from build123d import *

# Parameters (mm, degrees)
CROQUIS1_R              = 1.75
CROQUIS1_R_2            = 1.5
SALIENTE_EXTRUIR1_DEPTH = 2.5


with BuildPart() as part:
    # Croquis1 → Saliente-Extruir1 (new body)
    with BuildSketch(Plane(origin=(0, 0, 0), x_dir=(0, 0, -1), z_dir=(1, 0, 0))):
        with BuildLine():
            Line((95, 10), (90, 10))
            ThreePointArc((90, 10), (64.751798433, 28.463425825), (33.494108419, 27.311648705))
            ThreePointArc((33.494108419, 27.311648705), (20.033827629, 26.787261985), (6.785305839, 29.222587577))
            ThreePointArc((6.785305839, 29.222587577), (-24.970289012, 16.62782808), (-24.346472536, -17.528527464))
            ThreePointArc((-24.346472536, -17.528527464), (-24.321884003, -22.514223272), (-20, -25))
            ThreePointArc((-20, -25), (34.355278896, -56.609528466), (95, -40))
            Line((95, -40), (95, -35))
            Line((95, -35), (100, -35))
            Line((100, -35), (100, 5))
            Line((100, 5), (95, 5))
            Line((95, 5), (95, 10))
        make_face()
        with Locations((-12.730077402, 5.654698909)):
            Circle(CROQUIS1_R, mode=Mode.SUBTRACT)
        with Locations((-5.658477353, 12.726298958)):
            Circle(CROQUIS1_R, mode=Mode.SUBTRACT)
        with Locations((26.870057685, -19.798989873)):
            Circle(CROQUIS1_R, mode=Mode.SUBTRACT)
        with Locations((19.797157185, -26.871890373)):
            Circle(CROQUIS1_R, mode=Mode.SUBTRACT)
        with Locations((-20, -20)):
            Circle(CROQUIS1_R, mode=Mode.SUBTRACT)
        with Locations((90, -6.821183735)):
            Circle(CROQUIS1_R_2, mode=Mode.SUBTRACT)
        with Locations((90, -24.395183951)):
            Circle(CROQUIS1_R_2, mode=Mode.SUBTRACT)
        with Locations((44.87119885, -46.048776814)):
            Circle(CROQUIS1_R_2, mode=Mode.SUBTRACT)
        with Locations((44.87119885, 24.012524519)):
            Circle(CROQUIS1_R_2, mode=Mode.SUBTRACT)
        Polygon((-14.142135624, 0), (14.142135624, -28.284271247), (20.150710576, -22.275696296), (24.393351263, -26.518336983), (26.516504294, -24.395183951), (22.273863607, -20.152543264), (28.284271247, -14.142135624), (0, 14.142135624), (-6.01040764, 8.131727984), (-10.253048327, 12.374368671), (-12.374368671, 10.253048327), (-8.131727984, 6.01040764), align=None, mode=Mode.SUBTRACT)
    extrude(amount=SALIENTE_EXTRUIR1_DEPTH)


solid = part.part
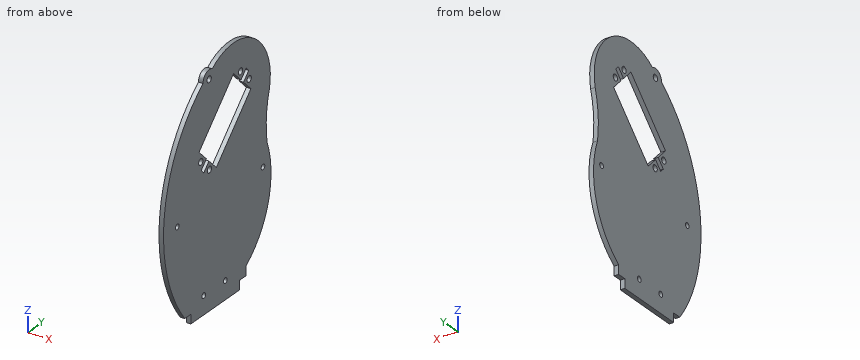
Read the model definition and answer for the solid it produces. Units are mm, in the model's axes. Coordinates: 2 decimals unless noted, no trailing zeros. Order: outer loops, then holes, each group sorted by start corner. A loop starts at its lowest first (then second) coordinate and runs counter-clockwise, first axis right, second up. Notation, with made-up numbers: M -30,-22.75 L 13,-22.75 A15 cw 13,4.25 Z; hole C -28.5,84 d9. An arc over 180 degrees is marked long. Put each result on its own line as item: value. Start each with the question number.
Item 1: Given pin 1 Ø3 at (y, z) = (-20, 20) entering from +X; pin 2 Ø0.8 at (x, y) = (1, -36.5) entering from -Z; pin 3 Ø0.8 at (x, z) = (0.5, -93) entering from +Y; pin 4 Ø1.2 at (x, z) = (0.5, -97.5) entering from -Y, each flat-ended and moving along its own axis, determine where each tip first touches the part or whether it passes through.
Item 2: Section A-A, the plane z = -4.5 is taken. Determine the outline of the cut face in (x, y), plus the area to 3 significant figures.
Item 3: Consider probe 1 along Z at (x, y) = (1, 6); probe 2 along Z at (x, y) = (0.8, 7); probe 3 along Z at (x, y) = (2.15, -20.5). Determine where each line is inside the solid, lowest interval first. Write a range as [from, to].
Item 4: Section B-B, the plane x = 1.6 is taken. Count the separate pieces of the cut face and the enclosed holes in it, plus the area to 3 significant figures.
Computed:
1. pin 1: passes through
1. pin 2: stops at z = -95
1. pin 3: stops at y = 10
1. pin 4: stops at y = -35
2. outline: M 0,-46.56 L 2.5,-46.56 L 2.5,-18.64 L 0,-18.64 Z; M 0,9.64 L 2.5,9.64 L 2.5,29.66 L 0,29.66 Z
2. area: 120 mm2
3. probe 1: z = [-95, -8.14], [8.14, 11.01], [14.45, 29.39]
3. probe 2: z = [-95, -7.14], [9.12, 11.61], [13.85, 29.17]
3. probe 3: z = [-100, -28.47], [-25.27, -22.62], [-6.36, 18.32], [21.68, 24.97]
4. separate pieces: 1
4. enclosed holes: 10
4. area: 8,300 mm2
